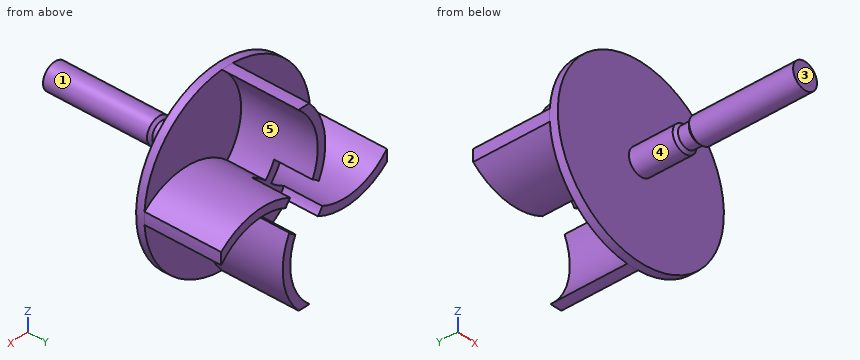
```python
from build123d import *

# Parameters (mm, degrees)
SKETCH1_R           = 33
BOSS_EXTRUDE1_DEPTH = 3
BOSS_EXTRUDE3_DEPTH = 28
CIRPATTERN2_COUNT   = 4
SKETCH4_R           = 8
CUT_EXTRUDE1_DEPTH  = 14
SKETCH5_R           = 4.75
BOSS_EXTRUDE4_DEPTH = 60


with BuildPart() as part:
    # Sketch1 → Boss-Extrude1 (new body)
    with BuildSketch(Plane(origin=(0, 0, 0), x_dir=(1, 0, 0), z_dir=(0, 1, 0))):
        with Locations(Location((0, 0, 0), (0, 0, 270))):
            Circle(SKETCH1_R)
    extrude(amount=BOSS_EXTRUDE1_DEPTH)

    # Sketch3 → Boss-Extrude3 (add)
    with BuildSketch(Plane(origin=(0, 3, 0), x_dir=(1, 0, 0), z_dir=(0, 1, 0))):
        with BuildLine():
            Line((1.076086957, 1.045005676), (-1.076086957, -1.045005676))
            ThreePointArc((-1.076086957, -1.045005676), (15.703563953, -8.46363111), (32.929819694, -2.151040426))
            ThreePointArc((32.929819694, -2.151040426), (32.999999926, 0.002211213), (32.929531131, 2.155453428))
            ThreePointArc((32.929531131, 2.155453428), (17.249059735, -5.463527063), (1.076086957, 1.045005676))
        make_face()
    boss_extrude3 = extrude(amount=BOSS_EXTRUDE3_DEPTH)

    # CirPattern2: Boss-Extrude3 ×4 about axis
    cirpattern2_axis = Axis((0, 0, 0), (0, 1, 0))
    for i in range(1, CIRPATTERN2_COUNT):
        add(boss_extrude3.rotate(cirpattern2_axis, i * 360 / CIRPATTERN2_COUNT))

    # Sketch4 → Cut-Extrude1 (cut)
    with BuildSketch(Plane(origin=(0, 31, 0), x_dir=(1, 0, 0), z_dir=(0, 1, 0))):
        Circle(SKETCH4_R)
    extrude(amount=-CUT_EXTRUDE1_DEPTH, mode=Mode.SUBTRACT)

    # Sketch5 → Boss-Extrude4 (add)
    with BuildSketch(Plane.XZ):
        with Locations(Location((0, 0, 0), (0, 0, 90))):
            Circle(SKETCH5_R)
    extrude(amount=BOSS_EXTRUDE4_DEPTH)

    # Sketch6 → Cut-Revolve1 (revolve, cut)
    with BuildSketch(Plane.XY, mode=Mode.PRIVATE) as cut_revolve1_sk:
        Polygon((-4.75, -16), (-3.75, -17), (-3.75, -21), (-4.75, -22), align=None)
    revolve(cut_revolve1_sk.sketch.rotate(Axis((0, 0, 0), (0, -1, 0)), 270), axis=Axis((0, 0, 0), (0, -1, 0)), mode=Mode.SUBTRACT)


solid = part.part
```
Verification items for the finished model (mm, model axes). Face numbers are marked on the shaded views. A direction names the side the tool comes from. Round coordinates to 2 decimals unless told otherwise and drop trailing zeros. Write each loop counter-clockwise with the first axis right and the second up, starting at its lowest first coordinate (ties: lowest second). Pieces come first, ordered by that corner, then holes. Notation, with made-up numbers: (66.5, 60.5) -> (94.5, 60.5) arc R26 ccw to (94.5, 78.5) -> close; hole circle Ø8 at (56.25, 14). An arc over 180 degrees is marked (long way). Write each question's results on one line, items separated by ' | '. Start each with the question number.
1. Cross-section at D-D (y = -50). Enter the section's corners in (x, z), then the cut area to 3 significant figures.
2. Cross-section at C-C (x = -16). Enter the section's corners in (y, z), then the cut area to 3 significant figures.
3. Depth check by flat-ended pin: P1, Ø1.5, axis at x = -20, z = -11.5, coming from the +Y side; P2, Ø4, axis at x = 25.5, z = -1, coming from the -Y side; P3, Ø7, axis at x = -2.5, z = -0.5, coming from the +Y side. Enter the tip coordinate at first touch or a pass-through.
4. Material ranges on probe 1 along Y at (x, z) = (11, 2); probe 2 along Z at (x, y) = (-16.5, 6.5); probe 3 along X at (y, z) = (17, -16.5), recorded low to high. Write a range as from..to.
5. Set-up check for the marked faces 4 and 5: record each of +Z, -Z, +X, -X, +Y, -Y from which the full face is reachable in a straight line by a thin tool's end or side.
6. Draft check along Z on the marked faces 1, 2 and 3. Enter one of: +Z half, -Z half, draft (parallel to the pull), parting line (faces both ways), or undercut.
7. Cross-section at A-A (y = 7.5). Enter the section's corners in (x, z), then the cut area to 3 significant figures.
8. Cross-section at B-B (z = -16.5). Enter the section's corners in (x, y), then the cut area to 3 significant figures.
Solutions:
1) outline: circle Ø9.5 at (0, 0) | area: 70.9 mm2
2) outline: (0, -28.86) -> (3, -28.86) -> (3, -8.47) -> (31, -8.47) -> (31, -5.47) -> (3, -5.47) -> (3, 28.86) -> (0, 28.86) -> close | area: 257 mm2
3) P1: stops at y = 3 | P2: stops at y = 0 | P3: stops at y = 17
4) probe 1: y = 0..3 | probe 2: z = -8.48..-5.48 | probe 3: x = 5.48..8.48
5) face 4: -Y | face 5: +Y
6) face 1: parting line | face 2: undercut | face 3: draft
7) outline: (-32.93, -2.15) arc R24.5 ccw to (-0.04, -2.12) arc R21.5 cw to (-2.16, -32.93) arc R33 ccw to (2.15, -32.93) arc R24.5 ccw to (2.12, -0.04) arc R21.5 cw to (32.93, -2.16) arc R33 ccw to (32.93, 2.15) arc R24.5 ccw to (0.04, 2.12) arc R21.5 cw to (2.16, 32.93) arc R33 ccw to (-2.15, 32.93) arc R24.5 ccw to (-2.12, 0.04) arc R21.5 cw to (-32.93, 2.16) arc R33 ccw to start | area: 432 mm2
8) outline: (-28.58, 0) -> (28.58, 0) -> (28.58, 3) -> (8.48, 3) -> (8.48, 31) -> (5.48, 31) -> (5.48, 3) -> (-28.58, 3) -> close | area: 255 mm2
